```python
from build123d import *

# Parameters (mm, degrees)
CYLINDER001_R     = 4
CYLINDER001_DEPTH = 10
BOX011_W          = 10
BOX011_H          = 8
BOX011_DEPTH      = 3
CYLINDER002_R     = 4
CYLINDER002_DEPTH = 10
PAD002_DEPTH      = 110
BOX010_W          = 117
BOX010_H          = 104
BOX010_DEPTH      = 18
CHAMFER002_SIZE   = 6.07
BOX009_W          = 120
BOX009_H          = 110
BOX009_DEPTH      = 20
CHAMFER001_SIZE   = 7.07


with BuildPart() as cylinder001:
    # Cylinder001 → Cylinder001 (new body)
    with BuildSketch(Plane(origin=(0, 0, 6), x_dir=(0, 0, -1), z_dir=(1, 0, 0))):
        Circle(CYLINDER001_R)
    extrude(amount=CYLINDER001_DEPTH)


with BuildPart() as cube011:
    # Box011 → Box011 (new body)
    with BuildSketch(Plane(origin=(0, -4, 3), x_dir=(1, 0, 0), z_dir=(0, 0, 1))):
        with Locations((5, 4)):
            Rectangle(BOX011_W, BOX011_H)
    extrude(amount=BOX011_DEPTH)


with BuildPart() as obj1:
    # Cylinder002 → Cylinder002 (new body)
    with BuildSketch(Plane(origin=(0, 0, 3), x_dir=(0, 0, -1), z_dir=(1, 0, 0))):
        Circle(CYLINDER002_R)
    extrude(amount=CYLINDER002_DEPTH)

    # Fusion002: union Cylinder001, Cube011
    add(cylinder001.part)
    add(cube011.part)


with BuildPart() as obj1_1:
    # Fusion002 placement: moved
    add(obj1.part.moved(Location((111, 55, 8))))


with BuildPart() as pad002:
    # Sketch002 → Pad002 (new body)
    with BuildSketch(Plane.XZ):
        Polygon((0, 0), (0, 23), (2.417397, 23), align=None)
    extrude(amount=-PAD002_DEPTH)


with BuildPart() as chamfer002:
    # Box010 → Box010 (new body)
    with BuildSketch(Plane(origin=(0, 3, 2), x_dir=(1, 0, 0), z_dir=(0, 0, 1))):
        with Locations((58.5, 52)):
            Rectangle(BOX010_W, BOX010_H)
    extrude(amount=BOX010_DEPTH)

    # Chamfer002
    chamfer002_edges = [chamfer002.edges().sort_by_distance(p)[0] for p in [
        (117, 55, 2),
        (58.5, 3, 2),
        (58.5, 107, 2),
    ]]
    chamfer(chamfer002_edges, length=CHAMFER002_SIZE)


with BuildPart() as obj2:
    # Box009 → Box009 (new body)
    with BuildSketch(Plane.XY):
        with Locations((60, 55)):
            Rectangle(BOX009_W, BOX009_H)
    extrude(amount=BOX009_DEPTH)

    # Chamfer001
    chamfer001_edges = [obj2.edges().sort_by_distance(p)[0] for p in [
        (120, 55, 0),
        (60, 0, 0),
        (60, 110, 0),
    ]]
    chamfer(chamfer001_edges, length=CHAMFER001_SIZE)

    # Cut006: cut Chamfer002
    add(chamfer002.part, mode=Mode.SUBTRACT)

    # Cut007: cut Pad002
    add(pad002.part, mode=Mode.SUBTRACT)

    # Cut008: cut obj1
    add(obj1_1.part, mode=Mode.SUBTRACT)


solid = obj2.part
```
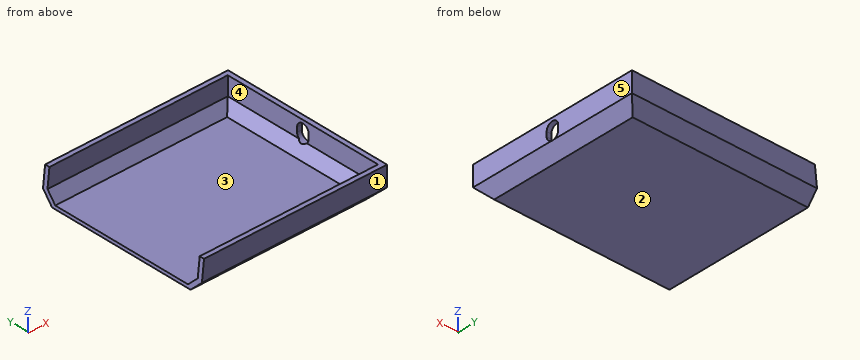
Design review of the part built by this model. Coordinates are the model's own, in mm. Face numbers are marked on the shaded views. A direction names the side the tool comes from. Give positions to 0.01 mm unless a question says otherwise; leave off trailing zeros. Loops run counter-clockwise (first coordinate to the right, second up) from the corner with the lowest first, then second, coordinate; pieces in that order, holes last. Notation, with made-up numbers: M 66,54 L 102,54 A19 ccw 102,63 Z; hole C -19.5,70.25 d9. An arc over 180 degrees is marked long. Return JSON: item names as keys, results as strings. Group by question number.
Item 1: For probe 1 along Y at (x, z) = (62, 15); probe 2 along Z at (x, y) = (46.5, 27); probe 3 along X at (y, z) = (74.5, 15.5), list the stretches that pass through material, from the lowest coordinate up.
Item 2: Mouldability with a two-part tool opening along Y and no side actions: class the marked faces 1, 2 and 3 as released by +Y, released by -Y, zero draft, split by the parting line, or undercut.
Item 3: Insertion check: pin 1 Ø1 at (x, z) = (103, 4.5) entering from +Y; pin 2 Ø6 at (x, y) = (69, 80.5) entering from +Z; pin 3 Ø1.5 at (y, z) = (36, 6) entering from -X. Each pin has a flat end and moves straight along its axis. Give the tip position at first contact, or say it passes through.
Item 4: Tool access review of the marked faces 4 and 5: name each direction out of +Z, -Z, +X, -X, +Y, -Y from which nothing blocks a thin tool from reaching the whole face with its end or side.
Item 5: We need section A-A (y = 68). Give the boundary of the cut face in (x, z), and give its area (3 significant figures).
Item 6: We need section B-B (x = 102). Give the boundary of the cut face in (y, z), and give its area (3 significant figures).
Output:
{
 "1": {"probe 1": "y = 0 to 3, 107 to 110", "probe 2": "z = 0 to 2", "probe 3": "x = 117 to 120"},
 "2": {"face 1": "released by -Y", "face 2": "zero draft", "face 3": "undercut"},
 "3": {"pin 1": "stops at y = 107.93", "pin 2": "stops at z = 2", "pin 3": "stops at x = 114.18"},
 "4": {"face 4": "+Z, -X", "face 5": "+Z, -Z, +X, +Y, -Y"},
 "5": {"outline": "M 0,0 L 112.93,0 L 120,7.07 L 120,20 L 117,20 L 117,8.07 L 110.93,2 L 0.21,2 Z", "area": "287 mm^2"},
 "6": {"outline": "M 0,7.07 L 7.07,0 L 102.93,0 L 110,7.07 L 110,20 L 107,20 L 107,8.07 L 100.93,2 L 9.07,2 L 3,8.07 L 3,20 L 0,20 Z", "area": "315 mm^2"}
}
